Autodesk Inventor part; units mm, degrees
ref_plane "YZ Plane" through (0, 0, 0) normal (1, 0, 0) x (0, 1, 0)
ref_plane "XZ Plane" through (0, 0, 0) normal (0, 1, 0) x (-1, 0, 0)
ref_plane "XY Plane" through (0, 0, 0) normal (0, 0, 1) x (1, 0, 0)
sketch "Szkic1" plane through (0, 0, 0) normal (0, 0, 1) x (1, 0, 0)
  line L0 (0, 0) -> (6.5, 0)
  line L1 (6.5, 0) -> (6.5, 15.75)
  line L2 (6.5, 15.75) -> (0, 15.75)
  line L3 (0, 15.75) -> (0, 0)
  point P0 (3.25, 12.5)
  dimension "d0" = 6.5
  dimension "d5" = 3.25
  dimension "d6" = 12.5
extrude "Wyciągnięcie proste1" add sketch "Szkic1" along normal mid plane 1
fillet "Zaokrąglenie1" radius 3.25 2 edges at (6.5, 15.75, 0) (0, 15.75, 0)
hole "Otwór1" at (3.25, 12.5, 0) direction (0, 0, -1) diameter 3 end through all both
properties part number "podporka_mala"
Input: part model. Units: mm. Frame: model coordinates. Give positions to 0.01 mm unless a question says otherwise; leave off trailing zeros. Order: outer loops, then holes, each group sorted by start corner. A loop starts at its lowest first (then second) coordinate and runs counter-clockwise, first axis right, second up. Notation, with made-up numbers: (80.25, 80.5) - (128.25, 80.5) arc R28 ccw to (128.25, 115.5) - close; hole circle Ø4 at (5, 82). An arc over 180 degrees is marked (long way). One line per item, written item: value.
1. Draft query along X for faces 1 (the face through (3, 8, 0.5)), 2 (the face through (0, 6, 0)), 3 (the face through (2.24, 13.61, -0.01)). Return one class per face: released by +X, released by -X, zero draft, split by the parting line, or undercut.
Determined:
face 1: zero draft
face 2: released by -X
face 3: undercut
2. Line query: probe 1 along Y at (x, z) = (3.25, 0.1); probe 2 along X at (y, z) = (12.5, -0.2); probe 3 along X at (y, z) = (13.75, -0.2). Output: solid intervals per line, ascending.
Determined:
probe 1: 0 to 11, 14 to 15.75
probe 2: 0 to 1.75, 4.75 to 6.5
probe 3: 0.25 to 2.42, 4.08 to 6.25
3. Cut plane B-B, the plane x = 2.5. Output: boundary loops of the cut face in (y, z), and give its area (3 significant figures).
Determined:
outline: (0, -0.5) - (11.2, -0.5) - (11.2, 0.5) - (0, 0.5) - close; (13.8, -0.5) - (15.66, -0.5) - (15.66, 0.5) - (13.8, 0.5) - close
area: 13.1 mm2
4. Cut plane C-C, the plane y = 12. Output: boundary loops of the cut face in (x, z).
Determined:
outline: (0, -0.5) - (1.84, -0.5) - (1.84, 0.5) - (0, 0.5) - close; (4.66, -0.5) - (6.5, -0.5) - (6.5, 0.5) - (4.66, 0.5) - close
